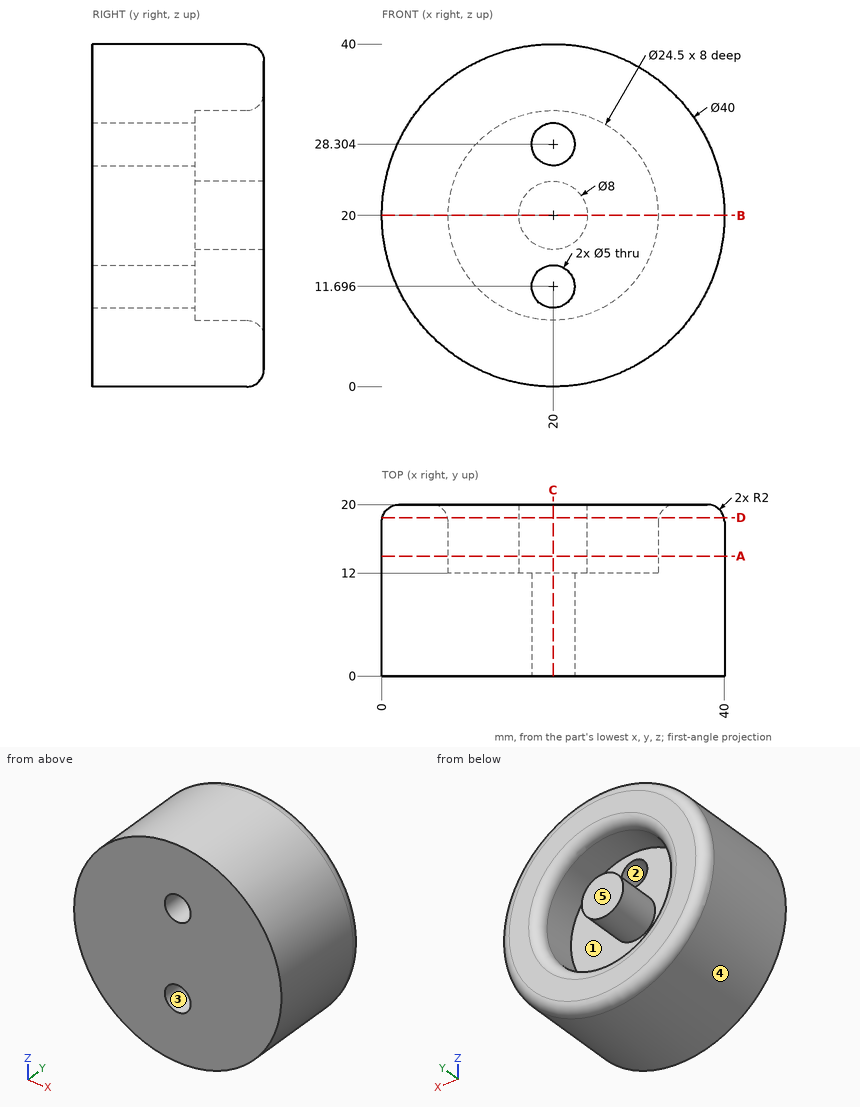
Geometry check sheet. Reference: drawing and pictorial views, mm from the part's lowest x, y, z. A direction names the side the tool comes from. Coordinates: 2 decimals unless noted, no trailing zeros. Order: outer loops, then holes, each group sorted by start corner. A loop starts at its lowest first (then second) coordinate and runs counter-clockwise, first axis right, second up.
Item 1: Access from +Z, -Z, +X, -X, +Y, -Y to the whole of each face (thin tool, end or side, straight path). Record for the marked faces 1 and 2.
Filled in:
face 1: +Y
face 2: +Y, -Y
Item 2: Section check A-A, the plane y = 14. Enter the section's corners in (x, z).
Filled in:
outline: circle Ø40 at (20, 20); circle Ø8 at (20, 20); hole circle Ø24.5 at (20, 20)
Item 3: Depth check by flat-ended pin: pin 1 (4 mm diameter, centred on y = 16, z = 12.5, fed in from -X); pin 2 (1.5 mm diameter, centred on y = 4.5, z = 30, fed in from +X); pin 3 (6.5 mm diameter, centred on x = 20, z = 28.3, fed in from +Y). Enter the tip coordinate at first touch or a pass-through.
Filled in:
pin 1: stops at x = 0.77
pin 2: stops at x = 37.73
pin 3: stops at y = 12
Item 4: Material ranges on L1, parallel to Z at x = 20, y = 14.55; L2, parallel to Z at x = 20, y = 7.5; L3, parallel to X at y = 13.75, z = 17 (1 decimal), recorded low to high.
Filled in:
L1: z = 0 to 7.75, 16 to 24, 32.25 to 40
L2: z = 0 to 9.2, 14.2 to 25.8, 30.8 to 40
L3: x = 0.2 to 8.1, 17.4 to 22.6, 31.9 to 39.8
Item 5: Release check for a two-part mould opening along X. For the marked faces 3, 4 and 5 record: +X half, -X half, draft (parallel to the pull), parting line (faces both ways), or undercut.
Filled in:
face 3: undercut
face 4: parting line
face 5: draft
Item 6: Section check B-B, the plane z = 20. Enter the section's corners in (x, y).
Filled in:
outline: (0, 0) - (40, 0) - (40, 18) arc R2 ccw to (38, 20) - (34.25, 20) arc R2 ccw to (32.25, 18) - (32.25, 12) - (24, 12) - (24, 20) - (16, 20) - (16, 12) - (7.75, 12) - (7.75, 18) arc R2 ccw to (5.75, 20) - (2, 20) arc R2 ccw to (0, 18) - close
Item 7: Section check C-C, the plane x = 20. Give the number of separate pieces and of enclosed holes in the cut face.
Filled in:
separate pieces: 3
enclosed holes: 0
Item 8: Section check D-D, the plane y = 18.5. Enter the section's corners in (x, z).
Filled in:
outline: circle Ø39.87 at (20, 20); circle Ø8 at (20, 20); hole circle Ø24.63 at (20, 20)
